The model under review builds one solid part; all positions refer to its coordinate system, in mm. Give positions to 0.01 mm unless a question says otherwise; leave off trailing zeros. Order: outer loops, then holes, each group sorted by start corner. A loop starts at its lowest first (then second) coordinate and runs counter-clockwise, first axis right, second up. Notation, with made-up numbers: (84, -33) - (100, -33) arc R13 ccw to (100, -17) - close; hole circle Ø2 at (26.5, 83). An arc over 180 degrees is marked (long way). Use CSV: the item, a comma, the result in double quotes. Start each with the question number.
```python
from build123d import *

# Parameters (mm, degrees)
SKETCH_W            = 327.5
SKETCH_H            = 196
SKETCH_W_2          = 311.5
SKETCH_H_2          = 178
PAD_DEPTH           = 2
SKETCH002_W         = 325.5
SKETCH002_H         = 194
SKETCH002_W_2       = 323.5
SKETCH002_H_2       = 192
PAD001_DEPTH        = 5
SKETCH005_R         = 0.95
POCKET_DEPTH        = 326.501
LINEARPATTERN_COUNT = 3
LINEARPATTERN_PITCH = 81
FILLET_R            = 0.25
FILLET001_R         = 1
FILLET002_R         = 0.25
FILLET003_R         = 1


with BuildPart() as part:
    # Sketch → Pad (new body)
    with BuildSketch(Plane.XY):
        with Locations((163.75, 98)):
            Rectangle(SKETCH_W, SKETCH_H)
        with Locations((163.75, 97)):
            Rectangle(SKETCH_W_2, SKETCH_H_2, mode=Mode.SUBTRACT)
    extrude(amount=PAD_DEPTH)

    # Sketch002 (on Face10 of Pad) → Pad001 (join)
    with BuildSketch(Plane.XY.offset(2)):
        with Locations((163.75, 98)):
            Rectangle(SKETCH002_W, SKETCH002_H)
        with Locations((163.75, 98)):
            Rectangle(SKETCH002_W_2, SKETCH002_H_2, mode=Mode.SUBTRACT)
    extrude(amount=PAD001_DEPTH)

    # Sketch005 (on Face12 of Pad001) → Pocket (cut, through all)
    with BuildSketch(Plane.YZ.offset(326.5)):
        with Locations((16, 3.5)):
            Circle(SKETCH005_R)
    pocket = extrude(amount=-POCKET_DEPTH, mode=Mode.SUBTRACT)

    # LinearPattern: Pocket ×3
    with Locations(*[(0, i * LINEARPATTERN_PITCH, 0) for i in range(1, LINEARPATTERN_COUNT)]):
        add(pocket, mode=Mode.SUBTRACT)

    # Fillet
    fillet_edges = [part.edges().sort_by_distance(p)[0] for p in [
        (2, 194, 4.5),
        (2, 2, 4.5),
        (325.5, 2, 4.5),
        (325.5, 194, 4.5),
    ]]
    fillet(fillet_edges, radius=FILLET_R)

    # Fillet001
    fillet001_edges = [part.edges().sort_by_distance(p)[0] for p in [
        (319.5, 186, 1),
        (319.5, 8, 1),
        (8, 186, 1),
        (8, 8, 1),
    ]]
    fillet(fillet001_edges, radius=FILLET001_R)

    # Fillet002
    fillet002_edges = [part.edges().sort_by_distance(p)[0] for p in [
        (163.75, 2, 2),
        (325.5, 98, 2),
        (163.75, 194, 2),
        (2, 98, 2),
        (2.073223, 193.926777, 2),
        (2.073223, 2.073223, 2),
        (325.426777, 2.073223, 2),
        (325.426777, 193.926777, 2),
    ]]
    fillet(fillet002_edges, radius=FILLET002_R)

    # Fillet003
    fillet003_edges = [part.edges().sort_by_distance(p)[0] for p in [
        (326.5, 1, 4.5),
        (326.5, 195, 4.5),
        (1, 1, 4.5),
        (1, 195, 4.5),
    ]]
    fillet(fillet003_edges, radius=FILLET003_R)


solid = part.part
```
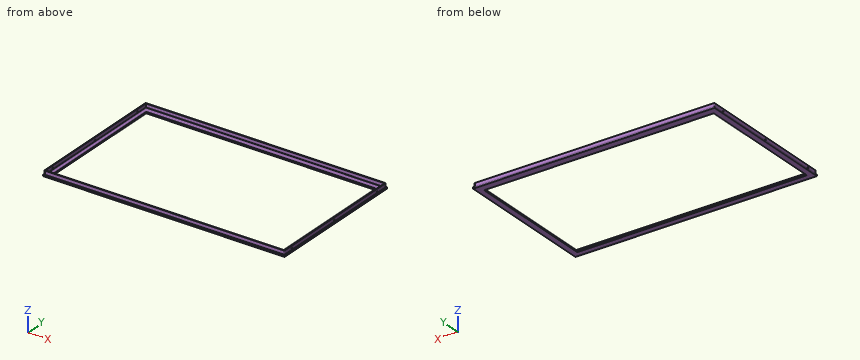
1. Consider section A-A (x = 105). Give the boundary of the cut face in (y, z).
2. Clearance check with flat-ended pins moving along their axes: pin 1 (2.5 mm diameter, centred on x = 235, z = 4.5, fed in from +Y); pin 2 (1.7 mm diameter, centred on y = 178, z = 3.5, fed in from +X); pin 3 (2.5 mm diameter, centred on y = 117, z = 5, fed in from -X); pin 4 (4 mm diameter, centred on x = 111.5, z = 3.5, fed in from -Y). State where each tip first meets the part, or that it passes through.
3. To check wall thickness, follow L1, parallel to Y at x = 206.5, z = 2.25; L2, parallel to X at y = 148.5, z = 2.25; L3, parallel to X at y = 24, z = 1.25. State the ranges of each line that lie inside material, in increasing order. Write a range as [from, to].
4. Consider section B-B (y = 124). Give the boundary of the cut face in (x, z).
Answers follow:
1,outline,"(0, 0) - (8, 0) - (8, 2) - (2.25, 2) arc R0.25 cw to (2, 2.25) - (2, 7) - (1, 7) - (1, 2) - (0, 2) - close; (186, 0) - (196, 0) - (196, 2) - (195, 2) - (195, 7) - (194, 7) - (194, 2.25) arc R0.25 cw to (193.75, 2) - (186, 2) - close"
2,pin 1,"stops at y = 195"
2,pin 2,"passes through"
2,pin 3,"stops at x = 1"
2,pin 4,"stops at y = 0"
3,L1,"y = [1, 2], [194, 195]"
3,L2,"x = [1, 2], [325.5, 326.5]"
3,L3,"x = [0, 8], [319.5, 327.5]"
4,outline,"(0, 0) - (8, 0) - (8, 2) - (2.25, 2) arc R0.25 cw to (2, 2.25) - (2, 7) - (1, 7) - (1, 2) - (0, 2) - close; (319.5, 0) - (327.5, 0) - (327.5, 2) - (326.5, 2) - (326.5, 7) - (325.5, 7) - (325.5, 2.25) arc R0.25 cw to (325.25, 2) - (319.5, 2) - close"
